Here's the drawing with two shaded views (mm, measured from the low corner). I have some questions. A direction names the side the tool comes from. Coordinates: 2 decimals unless noted, no trailing zeros. Write each loop counter-clockwise with the first axis right and the second up, starting at its lowest first coordinate (ties: lowest second). Pieces come first, ordered by that corner, then holes.
Item 1: If we section it at B-B (z = 27): Please give me the cut outline in (x, y) (3 decimals).
Item 2: If we section it at A-A (y = 38.1): Please give me the cut outline in (x, z) (3 decimals).
Item 3: If we section it at D-D (y = 14.5): Please give me the cut outline in (x, z).
Item 4: I'm going to push a flat-ended pin straight in: pin 1 Ø3 at (y, z) = (9, 28) entering from +X. Where does the tip first touch, or does it pass through?
Item 5: For the marked faces 4 and 5, which set-ups out of +Z, -Z, +X, -X, +Y, -Y let a thin tool reach every point of the face, with its end or its side?
Item 6: If we section it at C-C (x = 88.5): Please give me the cut outline in (y, z), then the cut area to 3 significant figures.
Item 7: We'd pull the mould along Z, two halves only. Please class the marked faces 1, 2 and 3: +Z half, -Z half, draft (parallel to the pull), parting line (faces both ways), or undercut.
Item 8: If I drill on line 1 (Y direction, x = 27, z = 38.1) (3 decimals); line 2 (X direction, y = 38.1, z = 19) (3 decimals), over which ranges is the centre line in solid material (lowest first)?
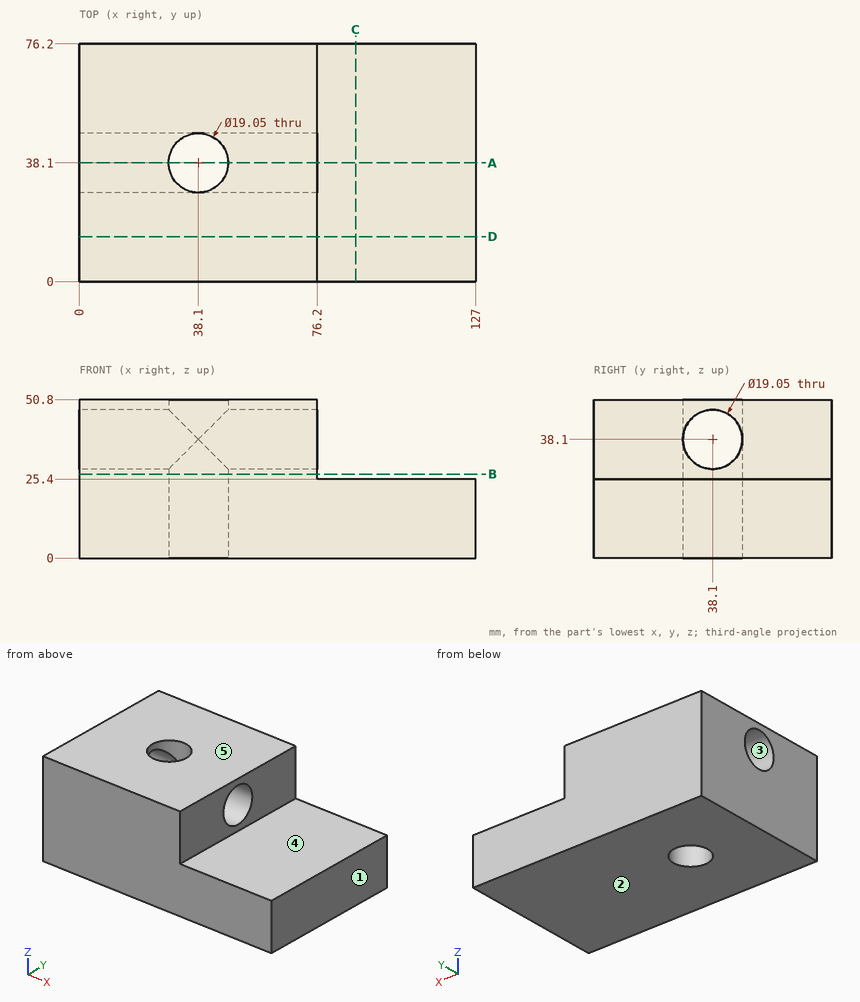
Answer list:
1. outline: (0, 0) - (76.2, 0) - (76.2, 76.2) - (0, 76.2) - close; hole circle Ø19.05 at (38.1, 38.1)
2. outline: (0, 0) - (28.575, 0) - (28.575, 28.575) - (0, 28.575) - close; (0, 47.625) - (28.575, 47.625) - (28.575, 50.8) - (0, 50.8) - close; (47.625, 0) - (127, 0) - (127, 25.4) - (76.2, 25.4) - (76.2, 28.575) - (47.625, 28.575) - close; (47.625, 47.625) - (76.2, 47.625) - (76.2, 50.8) - (47.625, 50.8) - close
3. outline: (0, 0) - (127, 0) - (127, 25.4) - (76.2, 25.4) - (76.2, 50.8) - (0, 50.8) - close
4. pin 1: stops at x = 76.2
5. face 4: +Z, +X, +Y, -Y
5. face 5: +Z, +X, -X, +Y, -Y
6. outline: (0, 0) - (76.2, 0) - (76.2, 25.4) - (0, 25.4) - close
6. area: 1,940 mm2
7. face 1: draft
7. face 2: -Z half
7. face 3: undercut
8. line 1: y = 0 to 28.575, 47.625 to 76.2
8. line 2: x = 0 to 28.575, 47.625 to 127
